Design review of the part built by this model. Coordinates are the model's own, in mm. Face numbers are marked on the shaded views. A direction names the side the tool comes from. Give positions to 0.01 mm unless a question says otherwise; leave off trailing zeros. Order: outer loops, then holes, each group sorted by start corner. A loop starts at its lowest first (then second) coordinate and runs counter-clockwise, first axis right, second up.
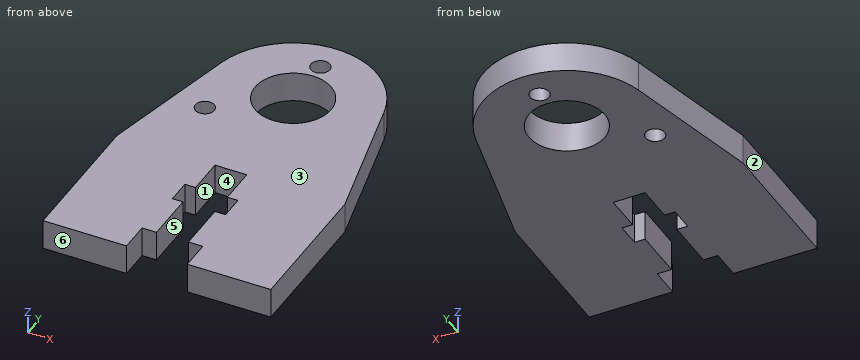
```python
from build123d import *

# Parameters (mm, degrees)
SKETCH6_R           = 5
BOSS_EXTRUDE5_DEPTH = 4
SKETCH10_R          = 1.25
CUT_EXTRUDE6_DEPTH  = 45.777226354
CUT_EXTRUDE7_DEPTH  = 45.777226354


with BuildPart() as part:
    # Sketch6 → Boss-Extrude5 (new body)
    with BuildSketch(Plane.XY):
        with BuildLine():
            Line((15, 0), (15, 15))
            Line((15, 15), (10.715935986, 33.483689987))
            ThreePointArc((10.715935986, 33.483689987), (0, 42), (-10.715935986, 33.483689987))
            Line((-10.715935986, 33.483689987), (-15, 15))
            Line((-15, 15), (-15, 0))
            Line((-15, 0), (-15, -4))
            Line((-15, -4), (-4, -4))
            Line((-4, -4), (-4, 0))
            Line((-4, 0), (4, 0))
            Line((4, 0), (4, -4))
            Line((4, -4), (15, -4))
            Line((15, -4), (15, 0))
        make_face()
        with Locations((0, 31)):
            Circle(SKETCH6_R, mode=Mode.SUBTRACT)
    extrude(amount=BOSS_EXTRUDE5_DEPTH)

    # Sketch10 → Cut-Extrude6 (cut, through all)
    with BuildSketch(Plane(origin=(0, 0, 0), x_dir=(-1, 0, 0), z_dir=(0, 0, -1))):
        with Locations((0, 38)):
            Circle(SKETCH10_R)
        with Locations((4.949747468, 44.949747468)):
            Circle(SKETCH10_R)
        with Locations((13.363961031, 46.363961031)):
            Circle(SKETCH10_R)
        with Locations((20.313708499, 41.414213562)):
            Circle(SKETCH10_R)
        with Locations((21.727922061, 33)):
            Circle(SKETCH10_R)
        with Locations((16.778174593, 26.050252532)):
            Circle(SKETCH10_R)
        with Locations((8.363961031, 24.636038969)):
            Circle(SKETCH10_R)
        with Locations((1.414213562, 29.585786438)):
            Circle(SKETCH10_R)
    extrude(amount=-CUT_EXTRUDE6_DEPTH, mode=Mode.SUBTRACT)

    # Sketch11 → Cut-Extrude7 (cut, through all)
    with BuildSketch(Plane.XY.offset(4)):
        Polygon((-2.1, 10), (-2.1, 15), (2.1, 15), (2.1, 10), (3.5, 10), (3.5, 6.8), (2.1, 6.8), (2.1, 0), (-2.1, 0), (-2.1, 6.8), (-3.5, 6.8), (-3.5, 10), align=None)
    extrude(amount=-CUT_EXTRUDE7_DEPTH, mode=Mode.SUBTRACT)


solid = part.part
```
1. For line 1 along Y through (x, z) = (0, 2.5); line 2 along X through (y, z) = (8.5, 2.75); line 3 along X through (y, z) = (13, 0.35), list the stretches that pass through material, from the lowest coordinate up.
Recorded:
line 1: y = 15 to 26, 36 to 36.75, 39.25 to 42
line 2: x = -15 to -3.5, 3.5 to 15
line 3: x = -15 to -2.1, 2.1 to 15
2. Take a section at B-B (x = 0). State the section outline as (y, z) points, then the cut area to 3 significant figures.
Recorded:
outline: (15, 0) - (26, 0) - (26, 4) - (15, 4) - close; (36, 0) - (36.75, 0) - (36.75, 4) - (36, 4) - close; (39.25, 0) - (42, 0) - (42, 4) - (39.25, 4) - close
area: 58.0 mm2
3. Take a section at C-C (z = 1.8). State the section outline as (x, y) points.
Recorded:
outline: (-15, -4) - (-4, -4) - (-4, 0) - (-2.1, 0) - (-2.1, 6.8) - (-3.5, 6.8) - (-3.5, 10) - (-2.1, 10) - (-2.1, 15) - (2.1, 15) - (2.1, 10) - (3.5, 10) - (3.5, 6.8) - (2.1, 6.8) - (2.1, 0) - (4, 0) - (4, -4) - (15, -4) - (15, 15) - (10.72, 33.48) arc R11 ccw to (-10.72, 33.48) - (-15, 15) - close; hole circle Ø2.5 at (-8.36, 24.64); hole circle Ø10 at (0, 31); hole circle Ø2.5 at (0, 38)
4. Take a section at A-A (y = 8.5). State the section outline as (x, z) points.
Recorded:
outline: (-15, 0) - (-3.5, 0) - (-3.5, 4) - (-15, 4) - close; (3.5, 0) - (15, 0) - (15, 4) - (3.5, 4) - close
5. Machinability: for the marked faces 5 and 6, which of the approach directions +Z, -Z, +X, -X, +Y, -Y give a long, thin tool a straight path to every point of the face, cutting with its end or side? Answer none if there is none.
Recorded:
face 5: +Z, -Z, -Y
face 6: +Z, -Z, +X, -X, -Y
6. For pin 1 (1.5 mm diameter, centred on y = 36, z = 1.5, fed in from -X); pin 2 (0.6 mm diameter, centred on x = -3, z = 2, fed in from -Y); pin 3 (1 mm diameter, centred on x = 0.5, z = 1, fed in from -Y); pin 4 (2 mm diameter, centred on x = -8.36, y = 24.64, fed in from -Z), all flat-tipped, find the tip position at first contact; note any pin that passes through.
Recorded:
pin 1: stops at x = -10.15
pin 2: stops at y = 0
pin 3: stops at y = 15
pin 4: passes through
7. Take a section at D-D (x = -8.75). State the section outline as (y, z) points, then the cut area to 3 significant figures.
Recorded:
outline: (-4, 0) - (23.45, 0) - (23.45, 4) - (-4, 4) - close; (25.82, 0) - (37.67, 0) - (37.67, 4) - (25.82, 4) - close
area: 157 mm2
8. Draft analysis for pull direction X (two halves, no side actions). For the marked faces 1, 2, 3 and 4, state which applies: pulls with the +X half, pulls with the -X half, needs draft (parallel to the pull), parting line crosses it, or undercut.
Recorded:
face 1: undercut
face 2: pulls with the -X half
face 3: needs draft
face 4: undercut
